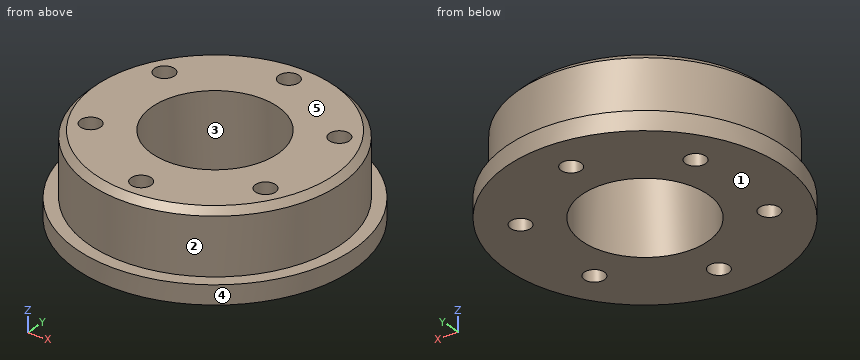
Autodesk Inventor part; units mm, degrees
ref_plane "YZ Plane" through (0, 0, 0) normal (1, 0, 0) x (0, 1, 0)
ref_plane "XZ Plane" through (0, 0, 0) normal (0, 1, 0) x (-1, 0, 0)
ref_plane "XY Plane" through (0, 0, 0) normal (0, 0, 1) x (1, 0, 0)
sketch "スケッチ1" plane through (0, 0, 0) normal (1, 0, 0) x (0, 1, 0)
  line L0 (10, 0) -> (10, -13)
  line L1 (22, -13) -> (22, -10)
  line L2 (22, -10) -> (20, -10)
  line L3 (20, -10) -> (20, 0)
  line L4 (20, 0) -> (10, 0)
  line L5 (0, -15.6) -> (0, 2.6)
  line L6 (22, -13) -> (10, -13)
  point P0 (0, 0)
  dimension "d0" = 20
  dimension "d1" = 2
  dimension "d2" = 10
  dimension "d3" = 3
  dimension "d4" = 10
revolve "回転1" add sketch "スケッチ1" angle 360 about axis through (0, 0, -10) along (0, 0, 1)
sketch "スケッチ2" plane through (0, 0, 0) normal (0, 0, 1) x (1, 0, 0)
  circle A0 centre (0, 0) radius 20
  circle A1 centre (0, 0) radius 16
  point P0 (0, 16)
  point P1 (-13.8564, 8)
  point P2 (-13.8564, -8)
  point P3 (0, -16)
  point P4 (13.8564, -8)
  point P5 (13.8564, 8)
  dimension "d8" = 4
  dimension "d11" = 360
hole "穴1" at (0, 16, 0) at (-13.8564, 8, 0) at (-13.8564, -8, 0) at (0, -16, 0) at (13.8564, -8, 0) at (13.8564, 8, 0) direction (0, 0, -1) diameter 3.2 end through all
chamfer "面取り1" distance 1 angle 45 1 edges at (0, -20, 0)
properties part number "base10" material "ABS プラスチック"
Verification items for the finished model (mm, model axes). Face numbers are marked on the shaded views. A direction names the side the tool comes from. Round coordinates to 2 decimals unless told otherwise and drop trailing zeros. Order: outer loops, then holes, each group sorted by start corner. A loop starts at its lowest first (then second) coordinate and runs counter-clockwise, first axis right, second up. Notation, with made-up numbers: (-5, 73.25) -> (41, 73.25) arc R18 ccw to (41, 105.25) -> close; hole circle Ø6 at (8, 73). An arc over 180 degrees is marked (long way). Put each result on its own line as item: value.
1) Set-up check for the marked faces 1 and 2: record each of +Z, -Z, +X, -X, +Y, -Y from which the full face is reachable in a straight line by a thin tool's end or side.
Final values:
face 1: -Z, +X, -X, +Y, -Y
face 2: +Z
2) Section check B-B (y = 0). Record the cut outline in (x, z).
Final values:
outline: (-22, -13) -> (-10, -13) -> (-10, 0) -> (-19, 0) -> (-20, -1) -> (-20, -10) -> (-22, -10) -> close; (10, -13) -> (22, -13) -> (22, -10) -> (20, -10) -> (20, -1) -> (19, 0) -> (10, 0) -> close
3) Section check C-C (z = -8.5). Record the cut outline in (x, y), then the cut area to 3 significant figures.
Final values:
outline: circle Ø40 at (0, 0); hole circle Ø3.2 at (-13.86, -8); hole circle Ø3.2 at (-13.86, 8); hole circle Ø20 at (0, 0); hole circle Ø3.2 at (0, -16); hole circle Ø3.2 at (0, 16); hole circle Ø3.2 at (13.86, -8); hole circle Ø3.2 at (13.86, 8)
area: 894 mm^2
4) Section check D-D (y = -7). Give the number of separate pieces and of enclosed holes in the cut face, then the cut area to 3 significant figures.
Final values:
separate pieces: 4
enclosed holes: 0
area: 248 mm^2
5) Section check A-A (x = 0). Record the cut outline in (y, z).
Final values:
outline: (-22, -13) -> (-17.6, -13) -> (-17.6, 0) -> (-19, 0) -> (-20, -1) -> (-20, -10) -> (-22, -10) -> close; (-14.4, -13) -> (-10, -13) -> (-10, 0) -> (-14.4, 0) -> close; (10, -13) -> (14.4, -13) -> (14.4, 0) -> (10, 0) -> close; (17.6, -13) -> (22, -13) -> (22, -10) -> (20, -10) -> (20, -1) -> (19, 0) -> (17.6, 0) -> close
6) Depth check by flat-ended pin: pin 1 (5 mm diameter, centred on y = 0, z = -1.5, fed in from +X); pin 2 (2.5 mm diameter, centred on x = 13.86, y = -8, fed in from +Z); pin 3 (4 mm diameter, centred on x = -4, z = -2, fed in from +Y); pin 4 (2 mm diameter, centred on x = 15, z = -8.5, fed in from -Y). Enter the tip coordinate at first touch or a pass-through.
Final values:
pin 1: stops at x = 20
pin 2: passes through
pin 3: stops at y = 19.9
pin 4: stops at y = -14.28
7) Mould release check, pull along X, two halves, no side actions. Record for the marked faces 3, 4 and 5: +X half, -X half, draft (parallel to the pull), parting line (faces both ways), or undercut.
Final values:
face 3: undercut
face 4: parting line
face 5: draft
8) Material ranges on line 1 (Y direction, x = 0, z = -6.5); line 2 (X direction, y = 0, z = -9); line 3 (X direction, y = -8, z = -7.25), recorded low to high.
Final values:
line 1: y = -20 to -17.6, -14.4 to -10, 10 to 14.4, 17.6 to 20
line 2: x = -20 to -10, 10 to 20
line 3: x = -18.33 to -15.46, -12.26 to -6, 6 to 12.26, 15.46 to 18.33
